from build123d import *

# Parameters (mm, degrees)
SKIZZE1_W                       = 75
SKIZZE1_H                       = 100
GRUNDPLATTE_DEPTH               = 4
SKIZZE2_R                       = 5
SKIZZE2_R_2                     = 3.5
SCHNITT_LINEAR_AUSTRAGEN1_DEPTH = 63.627869196


with BuildPart() as part:
    # Skizze1 → Grundplatte (new body)
    with BuildSketch(Plane.XY):
        Rectangle(SKIZZE1_W, SKIZZE1_H)
        with BuildLine():
            Line((25, 28), (-25, 28))
            ThreePointArc((-25, 28), (-27, 30), (-25, 32))
            Line((-25, 32), (25, 32))
            ThreePointArc((25, 32), (27, 30), (25, 28))
        make_face(mode=Mode.SUBTRACT)
        with BuildLine():
            Line((25, -28), (-25, -28))
            ThreePointArc((-25, -28), (-27, -30), (-25, -32))
            Line((-25, -32), (25, -32))
            ThreePointArc((25, -32), (27, -30), (25, -28))
        make_face(mode=Mode.SUBTRACT)
    extrude(amount=GRUNDPLATTE_DEPTH)

    # Skizze2 → Schnitt-Linear austragen1 (cut, through all)
    with BuildSketch(Plane.XY.offset(4)):
        with Locations((-28, 41)):
            Circle(SKIZZE2_R)
        with Locations((0, 41)):
            Circle(SKIZZE2_R)
        with Locations((28, 41)):
            Circle(SKIZZE2_R)
        with Locations((-14, 41)):
            Circle(SKIZZE2_R_2)
        with Locations((14, 41)):
            Circle(SKIZZE2_R_2)
        with Locations(Location((14, -41, 0), (0, 0, 180))):
            Circle(SKIZZE2_R_2)
        with Locations(Location((-14, -41, 0), (0, 0, 180))):
            Circle(SKIZZE2_R_2)
        with Locations(Location((28, -41, 0), (0, 0, 180))):
            Circle(SKIZZE2_R)
        with Locations(Location((0, -41, 0), (0, 0, 180))):
            Circle(SKIZZE2_R)
        with Locations(Location((-28, -41, 0), (0, 0, 180))):
            Circle(SKIZZE2_R)
        with BuildLine():
            Line((-33, -17.5), (-33, 17.5))
            ThreePointArc((-33, 17.5), (-28, 22.5), (-23, 17.5))
            Line((-23, 17.5), (-23, -17.5))
            ThreePointArc((-23, -17.5), (-28, -22.5), (-33, -17.5))
        make_face()
        with BuildLine():
            Line((5, 10), (5, -10))
            ThreePointArc((5, -10), (0, -15), (-5, -10))
            Line((-5, -10), (-5, 10))
            ThreePointArc((-5, 10), (0, 15), (5, 10))
        make_face()
        with BuildLine():
            Line((-9, 15), (-9, -15))
            ThreePointArc((-9, -15), (-14, -20), (-19, -15))
            Line((-19, -15), (-19, 15))
            ThreePointArc((-19, 15), (-14, 20), (-9, 15))
        make_face()
        with BuildLine():
            Line((9, 15), (9, -15))
            ThreePointArc((9, -15), (14, -20), (19, -15))
            Line((19, -15), (19, 15))
            ThreePointArc((19, 15), (14, 20), (9, 15))
        make_face()
        with BuildLine():
            Line((33, -17.5), (33, 17.5))
            ThreePointArc((33, 17.5), (28, 22.5), (23, 17.5))
            Line((23, 17.5), (23, -17.5))
            ThreePointArc((23, -17.5), (28, -22.5), (33, -17.5))
        make_face()
    extrude(amount=-SCHNITT_LINEAR_AUSTRAGEN1_DEPTH, mode=Mode.SUBTRACT)


solid = part.part
Could you check a few things on this model? Use its own coordinates, in mm. A direction names the side the tool comes from. Give positions to 0.01 mm unless a question says otherwise; leave off trailing zeros. Order: outer loops, then holes, each group sorted by start corner. A loop starts at its lowest first (then second) coordinate and runs counter-clockwise, first axis right, second up. Notation, with made-up numbers: (31, 87.25) - (73, 87.25) arc R24 cw to (73, 111.25) - close; hole circle Ø11 at (0, 16.5). An arc over 180 degrees is marked (long way). One line per question, with ' | ' between items. Start each with the question number.
Item 1: I'm going to push flat-ended pins straight in: pin 1 Ø13 at (x, y) = (28, -41) entering from +Z; pin 2 Ø9 at (x, y) = (-28, 41) entering from -Z. Where does each tip first touch, or does it pass through?
Item 2: I want a section at A-A on y = -41. Write out the boundary of the cut face in (x, z).
Item 3: I need wall thicknesses on probe 1 along X at (y, z) = (-41, 3.25); probe 2 along X at (y, z) = (15.5, 1); probe 3 along Y at (x, z) = (14, 2.45). Which ranges of each line are inside material? Lowest first, please. Write a range as [from, to].
Item 4: I want a section at C-C on y = 30. Write out the boundary of the cut face in (x, z), then the cut area to 3 significant figures.
Item 5: Thinking about a two-plate mould opening in Y: for faces 1 (the flat face through (8, 1, 0)), 2 (the flat face through (0, -32, 2)), 3 (the flat face through (-1, 50, 2)), which applies, pulls with the +Y half, pulls with the -Y half, needs draft (parallel to the pull), parting line crosses it, or undercut?
Item 6: I want a section at B-B on x = 20.5. Write out the boundary of the cut face in (y, z), then the cut area to 3 significant figures.
Item 7: For faces 4 (the flat face through (9, 0, 2)), 5 (the flat face through (8, 1, 4)), which set-ups out of +Z, -Z, +X, -X, +Y, -Y let a thin tool reach every point of the face, with its end or its side?
Item 8: I want a section at D-D on x = -14. Write out the boundary of the cut face in (y, z).
Verdict:
1) pin 1: z = 4 | pin 2: through
2) outline: (-37.5, 0) - (-33, 0) - (-33, 4) - (-37.5, 4) - close; (-23, 0) - (-17.5, 0) - (-17.5, 4) - (-23, 4) - close; (-10.5, 0) - (-5, 0) - (-5, 4) - (-10.5, 4) - close; (5, 0) - (10.5, 0) - (10.5, 4) - (5, 4) - close; (17.5, 0) - (23, 0) - (23, 4) - (17.5, 4) - close; (33, 0) - (37.5, 0) - (37.5, 4) - (33, 4) - close
3) probe 1: [-37.5, -33], [-23, -17.5], [-10.5, -5], [5, 10.5], [17.5, 23], [33, 37.5] | probe 2: [-37.5, -33], [-23, -18.97], [-9.03, 9.03], [18.97, 23], [33, 37.5] | probe 3: [-50, -44.5], [-37.5, -32], [-28, -20], [20, 28], [32, 37.5], [44.5, 50]
4) outline: (-37.5, 0) - (-27, 0) - (-27, 4) - (-37.5, 4) - close; (27, 0) - (37.5, 0) - (37.5, 4) - (27, 4) - close | area: 84.0 mm^2
5) face 1: needs draft | face 2: undercut | face 3: pulls with the +Y half
6) outline: (-50, 0) - (-32, 0) - (-32, 4) - (-50, 4) - close; (-28, 0) - (28, 0) - (28, 4) - (-28, 4) - close; (32, 0) - (50, 0) - (50, 4) - (32, 4) - close | area: 368 mm^2
7) face 4: +Z, -Z | face 5: +Z, +X, -X, +Y, -Y
8) outline: (-50, 0) - (-44.5, 0) - (-44.5, 4) - (-50, 4) - close; (-37.5, 0) - (-32, 0) - (-32, 4) - (-37.5, 4) - close; (-28, 0) - (-20, 0) - (-20, 4) - (-28, 4) - close; (20, 0) - (28, 0) - (28, 4) - (20, 4) - close; (32, 0) - (37.5, 0) - (37.5, 4) - (32, 4) - close; (44.5, 0) - (50, 0) - (50, 4) - (44.5, 4) - close
